from build123d import *

# Parameters (mm, degrees)
SKETCH1_R           = 16
BOSS_EXTRUDE1_DEPTH = 13.5
SKETCH2_W           = 7
SKETCH2_H           = 44
BOSS_EXTRUDE2_DEPTH = 4
FILLET1_R           = 2.54
SKETCH4_R           = 1.5
CUT_EXTRUDE1_DEPTH  = 31.368569278


with BuildPart() as part:
    # Sketch1 → Boss-Extrude1 (new body)
    with BuildSketch(Plane.XY):
        Circle(SKETCH1_R)
    extrude(amount=BOSS_EXTRUDE1_DEPTH)

    # Sketch2 → Boss-Extrude2 (add)
    with BuildSketch(Plane(origin=(0, 0, 0), x_dir=(-1, 0, 0), z_dir=(0, 0, -1))):
        Rectangle(SKETCH2_W, SKETCH2_H)
    extrude(amount=-BOSS_EXTRUDE2_DEPTH)

    # Fillet1
    fillet1_edges = [part.edges().sort_by_distance(p)[0] for p in [
        (-3.5, 22, 2),
        (3.5, -22, 2),
        (-3.5, -22, 2),
        (3.5, 22, 2),
    ]]
    fillet(fillet1_edges, radius=FILLET1_R)

    # Sketch4 → Cut-Extrude1 (cut, through all)
    with BuildSketch(Plane(origin=(0, 0, 0), x_dir=(-1, 0, 0), z_dir=(0, 0, -1))):
        with Locations((0, -19)):
            Circle(SKETCH4_R)
    cut_extrude1 = extrude(amount=-CUT_EXTRUDE1_DEPTH, mode=Mode.SUBTRACT)

    # Mirror1: Cut-Extrude1 across plane
    add(cut_extrude1.mirror(Plane.ZX), mode=Mode.SUBTRACT)


solid = part.part
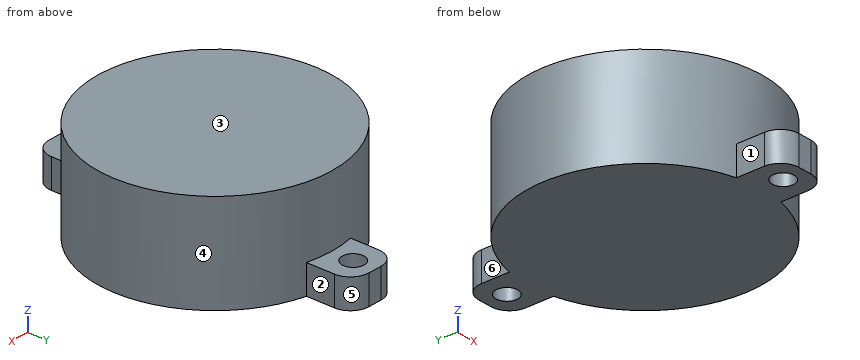
The model under review builds one solid part; all positions refer to its coordinate system, in mm. Face numbers are marked on the shaded views. A direction names the side the tool comes from. Coordinates: 2 decimals unless noted, no trailing zeros. Loops run counter-clockwise (first coordinate to the right, second up) from the corner with the lowest first, then second, coordinate; pieces in that order, holes last. Notation, with made-up numbers: (-8, 65.25) -> (17, 65.25) arc R21 cw to (17, 80.25) -> close; hole circle Ø8 at (79, -0.75). An arc over 180 degrees is marked (long way). Use a Markdown table: item, result. Add a question column.
1. To check wall thickness, follow line 1 (Y direction, x = 0, z = 1.3); line 2 (X direction, y = 19, z = 1.75); line 3 (Y direction, x = 0, z = 9.5). State the ranges of each line that lie inside material, in increasing order.
2. Add section A-A on z = 3.25. Write out the cut boundary in (x, y), plus the area to 3 significant figures.
3. Machinability: for the marked faces 1, 2 and 3, which of the approach directions +Z, -Z, +X, -X, +Y, -Y give a long, thin tool a straight path to every point of the face, cutting with its end or side? Answer none if there is none.
4. Add section C-C on y = 19. Write out the cut boundary in (x, z).
5. Add section B-B on x = 0. Write out the cut boundary in (y, z), plus the area to 3 significant figures.
6. Clearance check with flat-ended pins moving along their axes: pin 1 Ø4 at (x, y) = (0, 19) entering from +Z; pin 2 Ø3 at (y, z) = (8.5, 5) entering from +X; pin 3 Ø3 at (y, z) = (-18.5, 1.5) entering from +X. State where each tip first meets the part, or that it passes through.
7. Add section D-D on x = -10. Write out the cut boundary in (y, z).
8. Draft analysis for pull direction Y (two halves, no side actions). For the marked faces 4, 5 and 6, state which applies: pulls with the +Y half, pulls with the -Y half, needs draft (parallel to the pull), parting line crosses it, or undercut.
Returned:
| question | item | result |
|---|---|---|
| 1 | line 1 | y = -22 to -20.5, -17.5 to 17.5, 20.5 to 22 |
| 1 | line 2 | x = -3.5 to -1.5, 1.5 to 3.5 |
| 1 | line 3 | y = -16 to 16 |
| 2 | outline | (-3.5, -19.46) arc R2.54 ccw to (-0.96, -22) -> (0.96, -22) arc R2.54 ccw to (3.5, -19.46) -> (3.5, -15.61) arc R16 ccw to (3.5, 15.61) -> (3.5, 19.46) arc R2.54 ccw to (0.96, 22) -> (-0.96, 22) arc R2.54 ccw to (-3.5, 19.46) -> (-3.5, 15.61) arc R16 ccw to (-3.5, -15.61) -> close; hole circle Ø3 at (0, -19); hole circle Ø3 at (0, 19) |
| 2 | area | 870 mm² |
| 3 | face 1 | +Z, -Z, -X, -Y |
| 3 | face 2 | +Z, -Z, +X, +Y |
| 3 | face 3 | +Z, +X, -X, +Y, -Y |
| 4 | outline | (-3.5, 0) -> (-1.5, 0) -> (-1.5, 4) -> (-3.5, 4) -> close; (1.5, 0) -> (3.5, 0) -> (3.5, 4) -> (1.5, 4) -> close |
| 5 | outline | (-22, 0) -> (-20.5, 0) -> (-20.5, 4) -> (-22, 4) -> close; (-17.5, 0) -> (17.5, 0) -> (17.5, 4) -> (16, 4) -> (16, 13.5) -> (-16, 13.5) -> (-16, 4) -> (-17.5, 4) -> close; (20.5, 0) -> (22, 0) -> (22, 4) -> (20.5, 4) -> close |
| 5 | area | 456 mm² |
| 6 | pin 1 | stops at z = 4 |
| 6 | pin 2 | stops at x = 14.39 |
| 6 | pin 3 | stops at x = 3.5 |
| 7 | outline | (-12.49, 0) -> (12.49, 0) -> (12.49, 13.5) -> (-12.49, 13.5) -> close |
| 8 | face 4 | parting line crosses it |
| 8 | face 5 | pulls with the +Y half |
| 8 | face 6 | needs draft |
